from build123d import *

# Parameters (mm, degrees)
F1_DEPTH = 6
F3_DEPTH = 25


# Not quite as in the source:
# - a feature names something its author has since deleted; it is built from what else it names


with BuildPart() as f1:
    # F0 (on Top) → F1 (new body)
    with BuildSketch(Plane.XY):
        with BuildLine():
            ThreePointArc((104.075858604, -13.900203446), (104.7687099124, -6.9654449456), (105, 0))
            ThreePointArc((105, 0), (87.2496418331, 58.4166072277), (40, 97.0824391947))
            Line((40, 97.0824391947), (40, 80))
            Line((40, 80), (0, 80))
            Line((0, 80), (-40, 80))
            Line((-40, 80), (-40, 97.0824391947))
            ThreePointArc((-40, 97.0824391947), (-90.9326673974, 52.5), (-104.075858604, -13.900203446))
            Line((-104.075858604, -13.900203446), (-89.2820323028, -5.3589838486))
            Line((-89.2820323028, -5.3589838486), (-95.2820323028, 5.0333209968))
            Line((-95.2820323028, 5.0333209968), (-71.0910346562, 19))
            Line((-71.0910346562, 19), (-87.0824391947, 19))
            Line((-87.0824391947, 19), (-87.0824391947, 40))
            Line((-87.0824391947, 40), (-66.0824391947, 40))
            Line((-66.0824391947, 40), (-66.0824391947, 21.8917139379))
            Line((-66.0824391947, 21.8917139379), (-56.3108891325, 27.5333209968))
            Line((-56.3108891325, 27.5333209968), (-30.3108891325, -17.5))
            Line((-30.3108891325, -17.5), (-30.3108891325, 35))
            Line((-30.3108891325, 35), (30.3108891325, 35))
            Line((30.3108891325, 35), (30.3108891325, -17.5))
            Line((30.3108891325, -17.5), (56.3108891325, 27.5333209968))
            Line((56.3108891325, 27.5333209968), (66.0824391947, 21.8917139379))
            Line((66.0824391947, 21.8917139379), (66.0824391947, 40))
            Line((66.0824391947, 40), (87.0824391947, 40))
            Line((87.0824391947, 40), (87.0824391947, 19))
            Line((87.0824391947, 19), (71.0910346562, 19))
            Line((71.0910346562, 19), (95.2820323028, 5.0333209968))
            Line((95.2820323028, 5.0333209968), (89.2820323028, -5.3589838486))
            Line((89.2820323028, -5.3589838486), (104.075858604, -13.900203446))
        make_face()
        Polygon((-95.2820323028, 5.0333209968), (-89.2820323028, -5.3589838486), (-69.2820323028, -40), (-30.3108891325, -17.5), (-56.3108891325, 27.5333209968), (-66.0824391947, 21.8917139379), (-66.0824391947, 19), (-71.0910346562, 19), align=None)
        Polygon((0, -17.5), (30.3108891325, -17.5), (30.3108891325, 35), (-30.3108891325, 35), (-30.3108891325, -17.5), align=None)
        Polygon((69.2820323028, -40), (89.2820323028, -5.3589838486), (95.2820323028, 5.0333209968), (71.0910346562, 19), (66.0824391947, 19), (66.0824391947, 21.8917139379), (56.3108891325, 27.5333209968), (30.3108891325, -17.5), align=None)
        Polygon((-49.2820323028, -74.6410161514), (0, -75), (0, -17.5), (-30.3108891325, -17.5), (-69.2820323028, -40), align=None)
        Polygon((0, -75), (49.2820323028, -74.6410161514), (69.2820323028, -40), (30.3108891325, -17.5), (0, -17.5), align=None)
    extrude(amount=F1_DEPTH)

    # F2 (on face) → F3 (cut)
    with BuildSketch(Plane.XY.offset(6)):
        Polygon((-14.9996020609, -74.890738782), (0, -75), (14.9996020609, -74.890738782), (15.0003979391, -34.890738782), (-14.9996020609, -34.890738782), align=None)
    extrude(amount=-F3_DEPTH, mode=Mode.SUBTRACT)


solid = f1.part
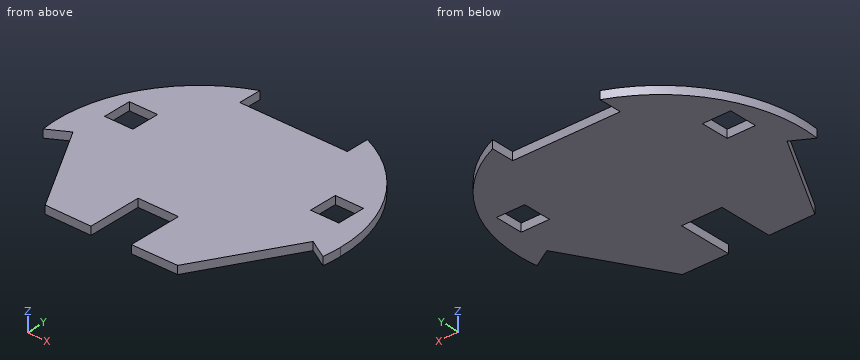
Could you check a few things on this model? Use its own coordinates, in mm. Give positions to 0.01 mm unless a question says otherwise; leave off trailing zeros. Order: outer loops, then holes, each group sorted by start corner. A loop starts at its lowest first (then second) coordinate and runs counter-clockwise, first axis right, second up.
Item 1: If we section it at D-D, the plane x = 82: Write out the boundary of the cut face in (y, z), plus the area to 3 significant figures.
Item 2: If we section it at A-A, the plane z = 4.75: Write out the boundary of the cut face in (x, y), plus the area to 3 significant figures.
Item 3: If we section it at C-C, the plane y = 26.5: Write out the boundary of the cut face in (x, z), plus the area to 3 significant figures.
Item 4: I'm going to push flat-ended pins straight in: pin 1 (1.8 mm diameter, centred on x = -74.5, z = 3, fed in from +Y); pin 2 (3 mm diameter, centred on y = 91.5, z = 1.5, fed in from -X); pin 3 (1.5 mm diameter, centred on x = 42, z = 1, fed in from -Y). Where does each tip first touch, or does it pass through?
Item 5: If we section it at B-B, the plane y = -58: Write out the boundary of the cut face in (x, z).
Item 6: I need wall thicknesses on line 1 (X direction, y = 21.5, z = 1.25); line 2 (X direction, y = 20, z = 3.75); line 3 (Y direction, x = -19, z = 1). Which ranges of each line are inside material? Lowest first, please.
Values:
1. outline: (-17.97, 0) - (19, 0) - (19, 6) - (-17.97, 6) - close; (40, 0) - (65.58, 0) - (65.58, 6) - (40, 6) - close
1. area: 375 mm2
2. outline: (-104.08, -13.9) - (-89.28, -5.36) - (-49.28, -74.64) - (-15, -74.89) - (-15, -34.89) - (15, -34.89) - (15, -74.89) - (49.28, -74.64) - (89.28, -5.36) - (104.08, -13.9) arc R105 ccw to (40, 97.08) - (40, 80) - (-40, 80) - (-40, 97.08) arc R105 ccw to start; hole (-87.08, 19) - (-66.08, 19) - (-66.08, 40) - (-87.08, 40) - close; hole (66.08, 19) - (87.08, 19) - (87.08, 40) - (66.08, 40) - close
2. area: 24,300 mm2
3. outline: (-101.6, 0) - (-87.08, 0) - (-87.08, 6) - (-101.6, 6) - close; (-66.08, 0) - (66.08, 0) - (66.08, 6) - (-66.08, 6) - close; (87.08, 0) - (101.6, 0) - (101.6, 6) - (87.08, 6) - close
3. area: 967 mm2
4. pin 1: stops at y = 74.89
4. pin 2: stops at x = -54.08
4. pin 3: stops at y = -74.7
5. outline: (-58.89, 0) - (-15, 0) - (-15, 6) - (-58.89, 6) - close; (15, 0) - (58.89, 0) - (58.89, 6) - (15, 6) - close
6. line 1: x = -102.78 to -87.08, -66.08 to 66.08, 87.08 to 102.78
6. line 2: x = -103.08 to -87.08, -66.08 to 66.08, 87.08 to 103.08
6. line 3: y = -74.86 to 80
